CAD build for the part. Positions are in the model's coordinates, mm. A direction names the side the tool comes from. Give positions to 0.01 mm unless a question says otherwise; leave off trailing zeros. Order: outer loops, then holes, each group sorted by start corner. A loop starts at its lowest first (then second) coordinate and runs counter-clockwise, first axis right, second up. Notation, with made-up numbers: (21.25, 46.25) -> (73.25, 46.25) arc R25 ccw to (73.25, 66.25) -> close; hole circle Ø11 at (-1.75, 6). An arc over 180 degrees is marked (long way). Answer as CSV lines item,"result".
```python
from build123d import *

# Parameters (mm, degrees)
F0_R     = 12.7
F1_DEPTH = 101.6
F3_W     = 12.7
F3_H     = 12.7


with BuildPart() as f1:
    # F0 (on Top) → F1 (new body)
    with BuildSketch(Plane.XY):
        Circle(F0_R)
    extrude(amount=F1_DEPTH)

    # F3 (on offset) → F4 (join, up to the next surface of F1)
    with BuildSketch(Plane.XZ.offset(25.4)):
        with Locations((0, 88.9)):
            Rectangle(F3_W, F3_H)
    extrude(until=Until.NEXT, dir=(0, 1, 0))


solid = f1.part
```
1) Band-saw the part on A-A, the plane x = 0. Write the cut outline in (y, z).
Data:
outline,"(-25.4, 82.55) -> (-12.7, 82.55) -> (-12.7, 0) -> (12.7, 0) -> (12.7, 101.6) -> (-12.7, 101.6) -> (-12.7, 95.25) -> (-25.4, 95.25) -> close"
2) Wall check: line 1 along Z through (x, y) = (-1.5, -20.5); line 2 along X through (y, z) = (-19.5, 85.5); line 3 along Y through (x, z) = (-11.5, 68). Give the ranges that are in metal, low to high. Write a range as [from, to].
Data:
line 1,"z = [82.55, 95.25]"
line 2,"x = [-6.35, 6.35]"
line 3,"y = [-5.39, 5.39]"
3) Band-saw the part on C-C, the plane y = -21. Write the cut outline in (x, z).
Data:
outline,"(-6.35, 82.55) -> (6.35, 82.55) -> (6.35, 95.25) -> (-6.35, 95.25) -> close"
4) Pin check, flat tips, straight feed: P1, Ø4, axis at y = -15.5, z = 90, coming from the +X side; P2, Ø6.5, axis at x = 1.5, y = -15.5, coming from the +Z side; P3, Ø5, axis at y = 6, z = 77, coming from the -X side; P4, Ø5, axis at x = 6, z = 80, coming from the -Y side. Stop position of each tip, or through.
Data:
P1,"stops at x = 6.35"
P2,"stops at z = 101.6"
P3,"stops at x = -12.21"
P4,"stops at y = -12.21"
5) Band-saw the part on B-B, the plane z = 81. Write the cut outline in (x, y).
Data:
outline,"circle Ø25.4 at (0, 0)"
6) Which spindle directions (+Z, -Z, +X, -X, +Y, -Y) get a long thin tool onto all of the face, cutting with end or side? Do faces 1 (the flat face through (-6.35, -18, 89)), 2 (the flat face through (6.35, -18, 89)), 3 (the flat face through (0, -25.4, 89)). Say none if no direction does.
Data:
face 1,"+Z, -Z, -X, -Y"
face 2,"+Z, -Z, +X, -Y"
face 3,"+Z, -Z, +X, -X, -Y"
7) Band-saw the part on D-D, the plane z = 93.5. Write the cut outline in (x, y), then the cut area to 3 significant figures.
Data:
outline,"(-6.35, -25.4) -> (6.35, -25.4) -> (6.35, -11) arc R12.7 ccw (long way) to (-6.35, -11) -> close"
area,"675 mm2"
